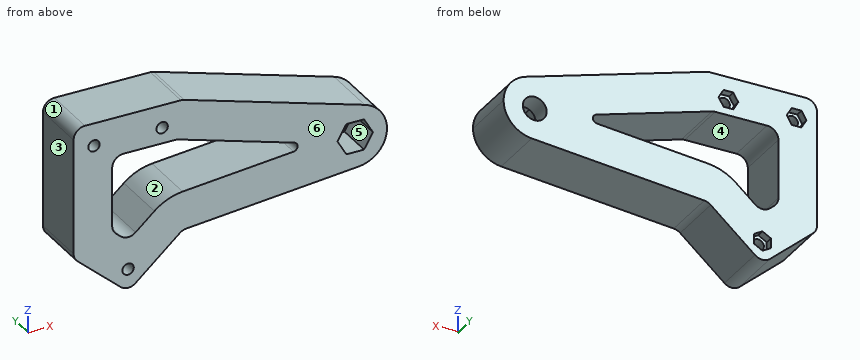
from build123d import *

# Parameters (mm, degrees)
F0_W      = 48
F0_H      = 58
F0_R      = 2.5
F0_W_2    = 90
F1_DEPTH  = 25
F3_DEPTH  = 16
F5_D      = 10.5
F7_DEPTH  = 25
F8_R      = 2.5
F9_DEPTH  = 3.5
F10_R     = 5
F12_DEPTH = 25.001
F13_R     = 5
F14_R     = 2


with BuildPart() as f1:
    # F0 (on Front) → F1 (new body)
    with BuildSketch(Plane.XZ):
        Rectangle(F0_W, F0_H)
        with Locations((-15, 19)):
            Circle(F0_R, mode=Mode.SUBTRACT)
        with Locations((15, 19)):
            Circle(F0_R, mode=Mode.SUBTRACT)
        with Locations((69, 0)):
            Rectangle(F0_W_2, F0_H)
        Polygon((24, -29), (-24, -29), (0, -50), align=None)
        with Locations((0, -40)):
            Circle(F0_R, mode=Mode.SUBTRACT)
    extrude(amount=F1_DEPTH)

    # F2 (on face) → F3 (cut)
    with BuildSketch(Plane.XZ.offset(25)):
        Polygon((96.102885683, -14.75), (103.897114317, -14.75), (107.7942286341, -8), (103.897114317, -1.25), (96.102885683, -1.25), (92.2057713659, -8), align=None)
    extrude(amount=-F3_DEPTH, mode=Mode.SUBTRACT)

    # F5 (through all)
    with Locations(Plane.XZ.offset(9)):
        with Locations((100.2942286341, -8)):
            Hole(F5_D / 2)

    # F6 (on face) → F7 (cut)
    with BuildSketch(Plane.XZ.offset(25)):
        with BuildLine():
            Line((114, 29), (24, 29))
            Line((24, 29), (104.2028684125, 5.1366169092))
            ThreePointArc((104.2028684125, 5.1366169092), (111.2810182281, 0.1938161532), (114, -7.9999999449))
            Line((114, -7.9999999449), (114, 29))
        make_face()
        with BuildLine():
            Line((114, -29), (114, -7.9999999449))
            ThreePointArc((114, -7.9999999449), (110.432692445, -17.222782676), (101.5877514086, -21.6445948114))
            Line((101.5877514086, -21.6445948114), (24, -29))
            Line((24, -29), (114, -29))
        make_face()
    extrude(amount=-F7_DEPTH, mode=Mode.SUBTRACT)

    # F8 (on face) → F9 (cut)
    with BuildSketch(Plane(origin=(0, 0, 0), x_dir=(-1, 0, 0), z_dir=(0, 1, 0))):
        Polygon((12.8349364905, 15.25), (17.1650635095, 15.25), (19.3301270189, 19), (17.1650635095, 22.75), (12.8349364905, 22.75), (10.6698729811, 19), align=None)
        with Locations((15, 19)):
            Circle(F8_R, mode=Mode.SUBTRACT)
        Polygon((-17.1650635095, 15.25), (-12.8349364905, 15.25), (-10.6698729811, 19), (-12.8349364905, 22.75), (-17.1650635095, 22.75), (-19.3301270189, 19), align=None)
        with Locations((-15, 19)):
            Circle(F8_R, mode=Mode.SUBTRACT)
        Polygon((-3.75, -42.1650635095), (0, -44.3301270189), (3.75, -42.1650635095), (3.75, -37.8349364905), (0, -35.6698729811), (-3.75, -37.8349364905), align=None)
        with Locations((0, -40)):
            Circle(F8_R, mode=Mode.SUBTRACT)
    extrude(amount=-F9_DEPTH, mode=Mode.SUBTRACT)

    # F10
    f10_edges = [f1.edges().sort_by_distance(p)[0] for p in [
        (-24, -12.5, 29),
        (24, -12.5, 29),
        (-24, -12.5, -29),
        (0, -12.5, -50),
        (24, -12.5, -29),
    ]]
    fillet(f10_edges, radius=F10_R)

    # F11 (on face) → F12 (cut, through all)
    with BuildSketch(Plane.XZ.offset(25)):
        with BuildLine():
            ThreePointArc((11.5911164871, -17.2687132217), (17.375962187, -13.6196897729), (24.0019026876, -11.9235988601))
            Line((24.0019026876, -11.9235988601), (83.1000312878, -6.3210304927))
            Line((83.1000312878, -6.3210304927), (21.5245542404, 12))
            Line((21.5245542404, 12), (-7, 12))
            Line((-7, 12), (-7, -21.2859401479))
            Line((-7, -21.2859401479), (0, -27.4109401479))
            Line((0, -27.4109401479), (11.5911164871, -17.2687132217))
        make_face()
    extrude(amount=-F12_DEPTH, mode=Mode.SUBTRACT)

    # F13
    f13_edges = [f1.edges().sort_by_distance(p)[0] for p in [
        (-7, -12.5, 12),
        (21.524554, -12.5, 12),
        (0, -12.5, -27.41094),
        (-7, -12.5, -21.28594),
    ]]
    fillet(f13_edges, radius=F13_R)

    # F14
    f14_edges = [f1.edges().sort_by_distance(p)[0] for p in [
        (83.100031, -12.5, -6.32103),
    ]]
    fillet(f14_edges, radius=F14_R)


solid = f1.part
Geometry: final body of the model. Coordinates: model frame, mm. Face numbers are marked on the shaded views. A direction names the side the tool comes from. Coordinates: 2 decimals unless noted, no trailing zeros. Order: outer loops, then holes, each group sorted by start corner. A loop starts at its lowest first (then second) coordinate and runs counter-clockwise, first axis right, second up. Notation, with made-up numbers: M 40,18 L 72,18 A17 ccw 72,26 Z; hole C 52,52.5 d1. An arc over 180 degrees is marked long. One line per question, with ' | ' between items. Start each with the question number.
Item 1: Draft query along Z for the marked faces 1, 2 and 3. Return one class per face: released by +Z, released by -Z, zero draft, split by the parting line, or undercut.
Item 2: Set-up query: the marked faces 4, 5 and 6. Return all of +Z, -Z, +X, -X, +Y, -Y with unobstructed straight access to the full face (end or side cutting, diameter ignored); none if empty.
Item 3: Cut plane D-D, the plane x = 15. Return the cut outline in (y, z) (3 decimals), then the cut area to 3 significant figures.
Item 4: Ray query, probe 1 along Z at (x, y) = (15, -17.5) (3 decimals); probe 2 along Z at (x, y) = (-1.5, -13.75); probe 3 along Z at (x, y) = (106.5, -9.5). Return the intervals inside material, ascending. Write a range as [from, to].
Item 5: Cut plane B-B, the plane x = 68. Return the cut outline in (y, z).
Item 6: Cut plane C-C, the plane z = -40. Return the cut outline in (x, y), then the cut area to 3 significant figures.
Item 7: Pin query (flat end, axial travel): pin 1 Ø4 at (x, y) = (73, -8.5) entering from +Z; pin 2 Ø5 at (x, y) = (19.5, -21) entering from -Z (3 decimals); pin 3 Ø1.5 at (y, z) = (-8.5, -39.5) entering from +X; pin 4 Ø3 at (x, z) = (15.5, -18) entering from +Y. Return the tip coordinate at first contact, or that it passes through.
Item 8: Cut plane A-A, the plane y = -13.75. Count the separate pieces of the cut face and the enclosed holes in it, then the cut area to 3 significant figures.
A:
1) face 1: released by +Z | face 2: undercut | face 3: zero draft
2) face 4: +Y, -Y | face 5: -Y | face 6: +Z, -Z, +X, -X, -Y
3) outline: M -25,-36.875 L 0,-36.875 L 0,-14.818 L -25,-14.818 Z; M -25,12 L 0,12 L 0,15.25 L -3.5,15.25 L -3.5,16.5 L -25,16.5 Z; M -25,21.5 L -3.5,21.5 L -3.5,22.75 L 0,22.75 L 0,29 L -25,29 Z | area: 843 mm2
4) probe 1: z = [-36.875, -14.818], [12, 16.5], [21.5, 29] | probe 2: z = [-48.13, -42], [-38, -25.54], [12, 29] | probe 3: z = [-20.22, -10.24], [-5.76, 4.22]
5) outline: M -25,-24.83 L 0,-24.83 L 0,-7.75 L -25,-7.75 Z; M -25,-1.83 L 0,-1.83 L 0,15.91 L -25,15.91 Z
6) outline: M -11.43,-25 L -2.5,-25 L -2.5,-3.5 L -3.75,-3.5 L -3.75,0 L -11.43,0 Z; M 2.5,-25 L 11.43,-25 L 11.43,0 L 3.75,0 L 3.75,-3.5 L 2.5,-3.5 Z | area: 438 mm2
7) pin 1: stops at z = 15.02 | pin 2: stops at z = -35.125 | pin 3: stops at x = 12.86 | pin 4: stops at y = 0
8) separate pieces: 1 | enclosed holes: 5 | area: 5,010 mm2
